from build123d import *

# Parameters (mm, degrees)
SKETCH1_R           = 17.96
BOSS_EXTRUDE1_DEPTH = 3
SKETCH2_W           = 150
SKETCH2_H           = 15
BOSS_EXTRUDE2_DEPTH = 30
BOSS_EXTRUDE3_START = 40
BOSS_EXTRUDE3_DEPTH = 40
FILLET1_R           = 2
SKETCH4_R           = 2
CUT_EXTRUDE1_DEPTH  = 4
SKETCH6_R           = 2
BOSS_EXTRUDE4_DEPTH = 40
SKETCH7_R           = 4.76
CUT_EXTRUDE4_DEPTH  = 30
SKETCH5_R           = 2
CUT_EXTRUDE6_DEPTH  = 60


with BuildPart() as part:
    # Sketch1 → Boss-Extrude1 (new body)
    with BuildSketch(Plane.XY):
        with BuildLine():
            Line((-75, 0), (-75, -75))
            Line((-75, -75), (-75, -90))
            Line((-75, -90), (75, -90))
            Line((75, -90), (75, -75))
            Line((75, -75), (75, 0))
            ThreePointArc((75, 0), (0, 75), (-75, 0))
        make_face()
        Circle(SKETCH1_R, mode=Mode.SUBTRACT)
    extrude(amount=BOSS_EXTRUDE1_DEPTH)

    # Sketch2 → Boss-Extrude2 (add)
    with BuildSketch(Plane(origin=(0, 0, 0), x_dir=(-1, 0, 0), z_dir=(0, 0, -1))):
        with Locations((0, -82.5)):
            Rectangle(SKETCH2_W, SKETCH2_H)
    extrude(amount=BOSS_EXTRUDE2_DEPTH)

    # Sketch3 → Boss-Extrude3 (add)
    with BuildSketch(Plane(origin=(0, 0, 0), x_dir=(-1, 0, 0), z_dir=(0, 0, -1)).offset(BOSS_EXTRUDE3_START)):
        with BuildLine():
            Line((75, 0), (75, -75))
            Line((75, -75), (72, -75))
            Line((72, -75), (72, 0))
            ThreePointArc((72, 0), (0, 72), (-72, 0))
            Line((-72, 0), (-72, -75))
            Line((-72, -75), (-75, -75))
            Line((-75, -75), (-75, 0))
            ThreePointArc((-75, 0), (0, 75), (75, 0))
        make_face()
    extrude(amount=-BOSS_EXTRUDE3_DEPTH)

    # Fillet1
    fillet1_edges = [part.edges().sort_by_distance(p)[0] for p in [
        (0, -75, 0),
        (72, -37.5, 0),
        (0, 72, 0),
        (-72, -37.5, 0),
    ]]
    fillet(fillet1_edges, radius=FILLET1_R)

    # Sketch4 → Cut-Extrude1 (cut)
    with BuildSketch(Plane.XY.offset(3)):
        with Locations((-67.5, -65)):
            Circle(SKETCH4_R)
        with Locations((67.5, -65)):
            Circle(SKETCH4_R)
        with Locations((67.5, -30)):
            Circle(SKETCH4_R)
        with Locations((67.5, 5)):
            Circle(SKETCH4_R)
        with Locations((-67.5, -30)):
            Circle(SKETCH4_R)
        with Locations((-67.5, 5)):
            Circle(SKETCH4_R)
    extrude(amount=-CUT_EXTRUDE1_DEPTH, mode=Mode.SUBTRACT)

    # Sketch6 → Boss-Extrude4 (add)
    with BuildSketch(Plane(origin=(0, 0, 0), x_dir=(-1, 0, 0), z_dir=(0, 0, -1))):
        with Locations(Location((43.16, -8.11, 0), (0, 0, 180))):
            Circle(SKETCH6_R)
        with Locations(Location((33.67, 17.57, 0), (0, 0, 180))):
            Circle(SKETCH6_R)
        with Locations(Location((33.67, 39.49, 0), (0, 0, 180))):
            Circle(SKETCH6_R)
    extrude(amount=BOSS_EXTRUDE4_DEPTH)

    # Sketch7 → Cut-Extrude4 (cut)
    with BuildSketch(Plane.ZY.offset(75)):
        with Locations((-23.57, 42.71)):
            Circle(SKETCH7_R)
    extrude(amount=-CUT_EXTRUDE4_DEPTH, mode=Mode.SUBTRACT)

    # Sketch5 → Cut-Extrude6 (cut)
    with BuildSketch(Plane.XY.offset(3)):
        with Locations((-45, 50)):
            Circle(SKETCH5_R)
        with Locations((45, 50)):
            Circle(SKETCH5_R)
    extrude(amount=-CUT_EXTRUDE6_DEPTH, mode=Mode.SUBTRACT)


solid = part.part
Geometry: final body of the model. Coordinates: model frame, mm. A direction names the side the tool comes from. Give positions to 0.01 mm unless a question says otherwise; leave off trailing zeros. Order: outer loops, then holes, each group sorted by start corner. A loop starts at its lowest first (then second) coordinate and runs counter-clockwise, first axis right, second up. Notation, with made-up numbers: (-8, 46.25) -> (39, 46.25) arc R17 cw to (39, 71.25) -> close; hole circle Ø4 at (27, 68). An arc over 180 degrees is marked (long way). Answer as a JSON object with one key per item and string values.
Q1. First-contact query: pin 1 (1.5 mm diameter, centred on x = 74, z = -36.5, fed in from -Y); pin 2 (5 mm diameter, centred on x = 32, z = -9, fed in from +Y); pin 3 (3.5 mm diameter, centred on x = -67.5, y = -65, fed in from -Z); pin 4 (1 mm diameter, centred on y = 29.5, z = -19, fed in from -X). Flat tips, straight axial feed; report the tip coordinate or a pass-through.
Entries:
{"pin 1": "stops at y = -75", "pin 2": "stops at y = 68.95", "pin 3": "passes through", "pin 4": "stops at x = -69.17"}
Q2. Section B-B (y = 5). State how many separate pieces and enclosed holes the cut face has, plus the area to 3 significant figures.
Entries:
{"separate pieces": "4", "enclosed holes": "0", "area": "564 mm^2"}
Q3. Material intervals for probe 1 along X at (y, z) = (-72.5, -2.5); probe 2 along Y at (x, z) = (-67.5, 0.6); probe 3 along Z at (x, y) = (-11, -56.5), sorted ascending.
Entries:
{"probe 1": "x = -75 to -72, 72 to 75", "probe 2": "y = -90 to -67, -63 to -32, -28 to 3, 7 to 32.69", "probe 3": "z = 0 to 3"}
Q4. Draft query along Y for faces 1 (the cylindrical face through (-66.577, -31.774, 1.521)), 2 (the cylindrical face through (1.65, 74.98, -18.8)), 3 (the cylindrical face through (-65.592, 5.601, 1.521)), 4 (the flat face through (-34, 18, -40)). Return one class per face: released by +Y, released by -Y, zero draft, split by the parting line, or undercut.
Entries:
{"face 1": "undercut", "face 2": "released by +Y", "face 3": "undercut", "face 4": "zero draft"}
Q5. Access query for faces 5 (the cylindrical face through (-1.583, 71.983, -21.266)), 6 (the flat face through (-1, -25, 3)), 7 (the flat face through (1, -82, -30)). Directions: +Z, -Z, +X, -X, +Y, -Y. A direction counts if a zero-diameter tool reaches every point of the face in a straight line with its end or side. Return the directions, or none.
Entries:
{"face 5": "-Z", "face 6": "+Z, +X, -X, +Y, -Y", "face 7": "-Z, +X, -X, -Y"}
Q6. Section A-A (y = -30). Output: boundary loops of the cut face in (x, z), plus the area to 3 significant figures.
Entries:
{"outline": "(-75, -40) -> (-72, -40) -> (-72, -2) arc R2 cw to (-70, 0) -> (-69.5, 0) -> (-69.5, 3) -> (-75, 3) -> close; (-65.5, 0) -> (65.5, 0) -> (65.5, 3) -> (-65.5, 3) -> close; (69.5, 0) -> (70, 0) arc R2 cw to (72, -2) -> (72, -40) -> (75, -40) -> (75, 3) -> (69.5, 3) -> close", "area": "668 mm^2"}
